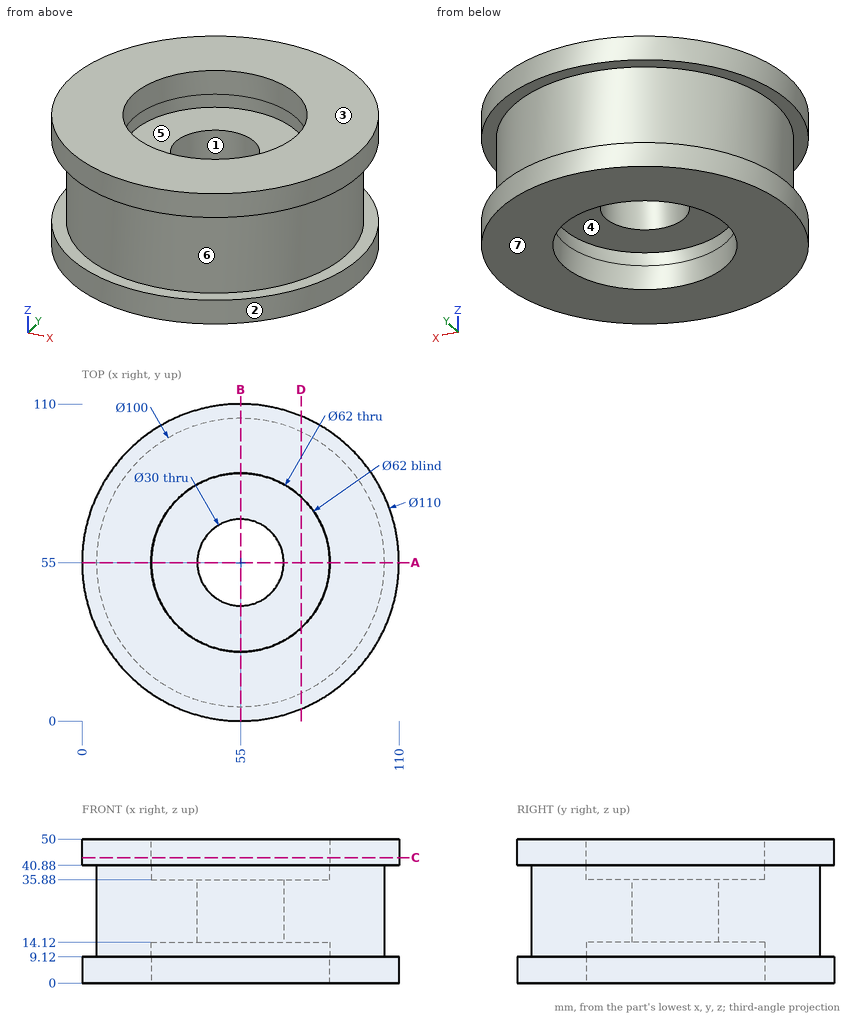
Source: three-view drawing plus pictorial views. Frame: mm from the lowest corner of the part. A direction names the side the tool comes from. Round coordinates to 2 decimals unless told otherwise and drop trailing zeros. Loops run counter-clockwise (first coordinate to the right, second up) from the corner with the lowest first, then second, coordinate; pieces in that order, holes last.
Item 1: Line query: L1, parallel to Y at x = 55, z = 19.75; L2, parallel to Y at x = 55, z = 48; L3, parallel to Z at x = 77, y = 66. Output: solid intervals per line, ascending.
Checked values:
L1: y = 5 to 40, 70 to 105
L2: y = 0 to 24, 86 to 110
L3: z = 14.12 to 35.88
Item 2: Section D-D, the plane x = 76. Output: boundary loops of the cut face in (y, z).
Checked values:
outline: (4.17, 0) - (32.2, 0) - (32.2, 14.12) - (77.8, 14.12) - (77.8, 0) - (105.83, 0) - (105.83, 9.12) - (100.38, 9.12) - (100.38, 40.88) - (105.83, 40.88) - (105.83, 50) - (77.8, 50) - (77.8, 35.88) - (32.2, 35.88) - (32.2, 50) - (4.17, 50) - (4.17, 40.88) - (9.62, 40.88) - (9.62, 9.12) - (4.17, 9.12) - close
Item 3: Section A-A, the plane y = 55. Output: boundary loops of the cut face in (x, z).
Checked values:
outline: (0, 0) - (24, 0) - (24, 14.12) - (40, 14.12) - (40, 35.88) - (24, 35.88) - (24, 50) - (0, 50) - (0, 40.88) - (5, 40.88) - (5, 9.12) - (0, 9.12) - close; (70, 14.12) - (86, 14.12) - (86, 0) - (110, 0) - (110, 9.12) - (105, 9.12) - (105, 40.88) - (110, 40.88) - (110, 50) - (86, 50) - (86, 35.88) - (70, 35.88) - close
Item 4: Mould query, pull axis Y, two halves, no side actions, for the marked faces 1, 2, 3 and 4. Classes: released by +Y, released by -Y, zero draft, split by the parting line, or undercut.
Checked values:
face 1: undercut
face 2: split by the parting line
face 3: zero draft
face 4: undercut
Item 5: Reachability of the marked faces 5, 6 and 7 from +Z, -Z, +X, -X, +Y, -Y: full face, straight path, thin tool, end or side. Return the list, or none.
Checked values:
face 5: +Z
face 6: none
face 7: -Z, +X, -X, +Y, -Y
Item 6: Contact query for flat-ended pins moving along their axis: P1, Ø24, axis at x = 55, y = 55, coming from the -Z side; P2, Ø2, axis at x = 60, z = 5, coming from the -Y side; P3, Ø10, axis at x = 64, z = 26, coming from the +Y side; P4, Ø1, axis at x = 91.5, y = 35.5, coming from the -Z side. Output: stop coordinate, or through.
Checked values:
P1: passes through
P2: stops at y = 0.15
P3: stops at y = 104.84
P4: stops at z = 0
Item 7: Section C-C, the plane z = 43.5. Output: boundary loops of the cut face in (x, y).
Checked values:
outline: circle Ø110 at (55, 55); hole circle Ø62 at (55, 55)
